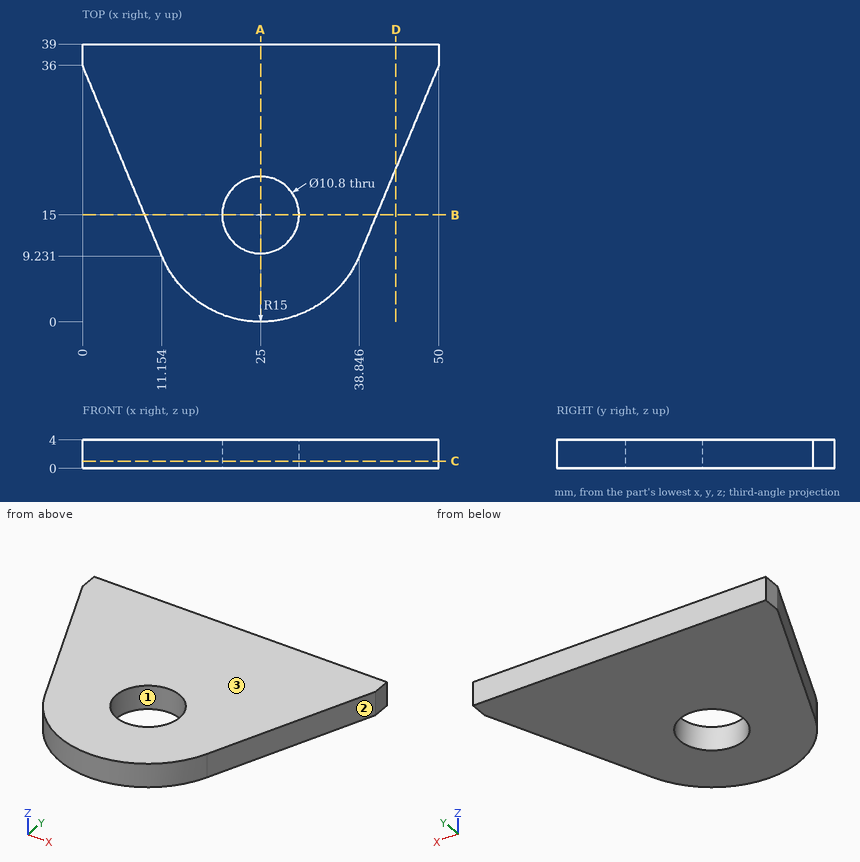
Geometry check sheet. Reference: drawing and pictorial views, mm from the part's lowest x, y, z. Give positions to 0.01 mm unless a question says otherwise; leave off trailing zeros. Write each loop counter-clockwise with the first axis right and the second up, starting at its lowest first coordinate (ties: lowest second). Pieces come first, ordered by that corner, then holes.
Item 1: Gauge pin test, flat end, axial feed: pin 1 (1 mm diameter, centred on x = 12.5, z = 2, fed in from -Y). Record the tip position at first contact, or that the pin passes through.
Item 2: Scan lines: L1, parallel to Y at x = 25, z = 3.25; L2, parallel to Y at x = 6.5, z = 3.6; L3, parallel to X at y = 17, z = 0.8. Record each from-to range of solid material in increasing order.
Item 3: Cross-section at C-C (z = 1). Enter the section's corners in (x, y).
Item 4: Cross-section at A-A (x = 25). Enter the section's corners in (y, z), and give its area (3 significant figures).
Item 5: Cross-section at D-D (x = 44). Enter the section's corners in (y, z), and give its area (3 significant figures).
Item 6: Cross-section at B-B (y = 15). Enter the section's corners in (x, z).
Item 7: Draft check along Y on the marked faces 1, 2 and 3. Enter one of: released by +Y, released by -Y, zero draft, split by the parting line, or undercut.
Report:
1. pin 1: stops at y = 6
2. L1: y = 0 to 9.6, 20.4 to 39
2. L2: y = 20.4 to 39
2. L3: x = 7.92 to 19.98, 30.02 to 42.08
3. outline: (0, 36) - (11.15, 9.23) arc R15 ccw to (38.85, 9.23) - (50, 36) - (50, 39) - (0, 39) - close; hole circle Ø10.8 at (25, 15)
4. outline: (0, 0) - (9.6, 0) - (9.6, 4) - (0, 4) - close; (20.4, 0) - (39, 0) - (39, 4) - (20.4, 4) - close
4. area: 113 mm2
5. outline: (21.6, 0) - (39, 0) - (39, 4) - (21.6, 4) - close
5. area: 69.6 mm2
6. outline: (8.75, 0) - (19.6, 0) - (19.6, 4) - (8.75, 4) - close; (30.4, 0) - (41.25, 0) - (41.25, 4) - (30.4, 4) - close
7. face 1: undercut
7. face 2: released by -Y
7. face 3: zero draft
